from build123d import *

# Parameters (mm, degrees)
EXTRUDE_1_DEPTH     = 3
SKETCH_2_R          = 3
CUT_EXTRUDE_1_DEPTH = 3
EXTRUDE_2_DEPTH     = 5


with BuildPart() as part:
    # 草图1 → 凸台-拉伸1 (new body)
    with BuildSketch(Plane(origin=(0, 0, 0), x_dir=(1, 0, 0), z_dir=(0, 1, 0))):
        Polygon((55, 0), (285, 0), (285, 20), (320, 20), (320, 55), (320, 285), (320, 320), (285, 320), (285, 340), (55, 340), (55, 320), (20, 320), (20, 285), (20, 55), (20, 20), (55, 20), align=None)
    extrude(amount=EXTRUDE_1_DEPTH)

    # 草图2 → 切除-拉伸1 (cut)
    with BuildSketch(Plane(origin=(0, 3, 0), x_dir=(1, 0, 0), z_dir=(0, 1, 0))):
        with Locations(Location((75, 330, 0), (0, 0, 270))):
            Circle(SKETCH_2_R)
        with Locations(Location((265, 330, 0), (0, 0, 90))):
            Circle(SKETCH_2_R)
        with Locations(Location((265, 10, 0), (0, 0, 270))):
            Circle(SKETCH_2_R)
        with Locations(Location((75, 10, 0), (0, 0, 90))):
            Circle(SKETCH_2_R)
    extrude(amount=-CUT_EXTRUDE_1_DEPTH, mode=Mode.SUBTRACT)

    # 草图3 → 凸台-拉伸2 (add)
    # profile 1 of 4: a face of its own
    with BuildSketch(Plane(origin=(0, 3, 0), x_dir=(1, 0, 0), z_dir=(0, 1, 0))):
        Polygon((111.431457505, 228.568542495), (111.431457505, 204.568542495), (120.431457505, 204.568542495), (120.431457505, 219.568542495), (138.38115839, 219.568542495), (138.38115839, 228.568542495), align=None)
        Polygon((113.431457505, 226.568542495), (113.431457505, 206.568542495), (118.431457505, 206.568542495), (118.431457505, 221.568542495), (136.38115839, 221.568542495), (136.38115839, 226.568542495), align=None, mode=Mode.SUBTRACT)
    # profile 2 of 4: a face of its own
    with BuildSketch(Plane(origin=(0, 3, 0), x_dir=(1, 0, 0), z_dir=(0, 1, 0))):
        Polygon((228.568542495, 228.568542495), (204.568542495, 228.568542495), (204.568542495, 219.568542495), (219.568542495, 219.568542495), (219.568542495, 201.61884161), (228.568542495, 201.61884161), align=None)
        Polygon((226.568542495, 226.568542495), (206.568542495, 226.568542495), (206.568542495, 221.568542495), (221.568542495, 221.568542495), (221.568542495, 203.61884161), (226.568542495, 203.61884161), align=None, mode=Mode.SUBTRACT)
    # profile 3 of 4: a face of its own
    with BuildSketch(Plane(origin=(0, 3, 0), x_dir=(1, 0, 0), z_dir=(0, 1, 0))):
        Polygon((228.568542495, 111.431457505), (228.568542495, 135.431457505), (219.568542495, 135.431457505), (219.568542495, 120.431457505), (201.61884161, 120.431457505), (201.61884161, 111.431457505), align=None)
        Polygon((226.568542495, 113.431457505), (226.568542495, 133.431457505), (221.568542495, 133.431457505), (221.568542495, 118.431457505), (203.61884161, 118.431457505), (203.61884161, 113.431457505), align=None, mode=Mode.SUBTRACT)
    # profile 4 of 4: a face of its own
    with BuildSketch(Plane(origin=(0, 3, 0), x_dir=(1, 0, 0), z_dir=(0, 1, 0))):
        Polygon((111.431457505, 111.431457505), (135.431457505, 111.431457505), (135.431457505, 120.431457505), (120.431457505, 120.431457505), (120.431457505, 138.38115839), (111.431457505, 138.38115839), align=None)
        Polygon((113.431457505, 113.431457505), (133.431457505, 113.431457505), (133.431457505, 118.431457505), (118.431457505, 118.431457505), (118.431457505, 136.38115839), (113.431457505, 136.38115839), align=None, mode=Mode.SUBTRACT)
    extrude(amount=EXTRUDE_2_DEPTH)


solid = part.part
Geometry: final body of the model. Coordinates: model frame, mm. Give positions to 0.01 mm unless a question says otherwise; leave off trailing zeros. Write each loop counter-clockwise with the first axis right and the second up, starting at its lowest first coordinate (ties: lowest second). Pieces come first, ordered by that corner, then holes. Notation, with made-up numbers: (40.25, 54.5) -> (73.25, 54.5) arc R10 ccw to (73.25, 67.5) -> close; hole circle Ø8 at (40.25, 36.5). An arc over 180 degrees is marked (long way). Answer in a Markdown table with one row per item.
(1) Pin query (flat end, axial travel): pin 1 (1.5 mm diameter, centred on x = 215, y = 6.5, fed in from -Z); pin 2 (8 mm diameter, centred on x = 281, z = -76.5, fed in from -Y); pin 3 (1.5 mm diameter, centred on x = 213, y = 6.5, fed in from +Z); pin 4 (4 mm diameter, centred on y = 6, z = -128, fed in from +X). Return the tip coordinate at first contact, or that it passes through.
Answers below:
| item | result |
|---|---|
| pin 1 | z = -228.57 |
| pin 2 | y = 0 |
| pin 3 | z = -111.43 |
| pin 4 | x = 228.57 |
(2) Ray query, line 1 along Z through (x, y) = (265, 2.2); line 2 along X through (y, z) = (2.05, -10); line 3 along Z through (x, y) = (222, 4.25). Return the intervals inside material, ascending. Write a range as [from, to].
Answers below:
| item | result |
|---|---|
| line 1 | [-340, -333], [-327, -13], [-7, 0] |
| line 2 | [55, 72], [78, 262], [268, 285] |
| line 3 | [-228.57, -226.57], [-203.62, -201.62], [-135.43, -133.43], [-113.43, -111.43] |
(3) Section query A-A on y = 1.5. Return loops of the section in (x, z), then the cut area to 3 significant figures.
Answers below:
| item | result |
|---|---|
| outline | (20, -320) -> (55, -320) -> (55, -340) -> (285, -340) -> (285, -320) -> (320, -320) -> (320, -20) -> (285, -20) -> (285, 0) -> (55, 0) -> (55, -20) -> (20, -20) -> close; hole circle Ø6 at (75, -330); hole circle Ø6 at (75, -10); hole circle Ø6 at (265, -330); hole circle Ø6 at (265, -10) |
| area | 99,100 mm^2 |
(4) Section query B-B on x = 154. Return loops of the section in (y, z).
Answers below:
| item | result |
|---|---|
| outline | (0, -340) -> (3, -340) -> (3, 0) -> (0, 0) -> close |
(5) Section query C-C on z = -35. Return loops of the section in (x, y), then the cut area to 3 significant figures.
Answers below:
| item | result |
|---|---|
| outline | (20, 0) -> (320, 0) -> (320, 3) -> (20, 3) -> close |
| area | 900 mm^2 |
(6) Draft query along Z for faces 1 (the flat face through (220, 3, -117)), 2 (the flat face through (120, 8, -122)). Return one class per face: +Z half, -Z half, draft (parallel to the pull), parting line (faces both ways), or undercut.
Answers below:
| item | result |
|---|---|
| face 1 | undercut |
| face 2 | draft |
